from build123d import *

# Parameters (mm, degrees)
SKETCH_1_W          = 195
SKETCH_1_H          = 50
EXTRUDE_1_DEPTH     = 4
SKETCH_5_W          = 195
SKETCH_5_H          = 50
EXTRUDE_2_DEPTH     = 4
SKETCH_2_R          = 1.5
CUT_EXTRUDE_1_DEPTH = 124.074164633
SKETCH_4_W          = 20
SKETCH_4_H          = 14
CUT_EXTRUDE_3_DEPTH = 124.074164633
FILLET_1_R          = 1.5
SKETCH_6_W          = 23
SKETCH_6_H          = 23
CUT_EXTRUDE_4_DEPTH = 124.074164633
FILLET_2_R          = 5
SKETCH_7_W          = 15
SKETCH_7_H          = 15
EXTRUDE_3_DEPTH     = 4
SKETCH_3_R          = 1.5
CUT_EXTRUDE_2_DEPTH = 124.074164633
SKETCH_8_R          = 1.5
CUT_EXTRUDE_5_DEPTH = 124.074164633
SKETCH_9_W          = 165
SKETCH_9_H          = 13
CUT_EXTRUDE_6_DEPTH = 124.074164633
FILLET_3_R          = 20


with BuildPart() as part:
    # 草图1 → 凸台-拉伸1 (new body)
    with BuildSketch(Plane.XY):
        Rectangle(SKETCH_1_W, SKETCH_1_H)
    extrude(amount=EXTRUDE_1_DEPTH)

    # 草图5 → 凸台-拉伸2 (add)
    with BuildSketch(Plane.XY.offset(4)):
        with Locations((0, 50)):
            Rectangle(SKETCH_5_W, SKETCH_5_H)
    extrude(amount=-EXTRUDE_2_DEPTH)

    # 草图2 → 切除-拉伸1 (cut, through all)
    with BuildSketch(Plane.XY.offset(4)):
        with Locations((-47.5, -3)):
            Circle(SKETCH_2_R)
        with Locations((-47.5, 9)):
            Circle(SKETCH_2_R)
        with Locations((47.5, 9)):
            Circle(SKETCH_2_R)
        with Locations((47.5, -3)):
            Circle(SKETCH_2_R)
    extrude(amount=-CUT_EXTRUDE_1_DEPTH, mode=Mode.SUBTRACT)

    # 草图4 → 切除-拉伸3 (cut, through all)
    with BuildSketch(Plane.XY.offset(4)):
        with Locations((47.5, 25)):
            Rectangle(SKETCH_4_W, SKETCH_4_H)
        with Locations((-47.5, 25)):
            Rectangle(SKETCH_4_W, SKETCH_4_H)
    extrude(amount=-CUT_EXTRUDE_3_DEPTH, mode=Mode.SUBTRACT)

    # 圆角1
    fillet_1_edges = [part.edges().sort_by_distance(p)[0] for p in [
        (37.5, 18, 2),
        (37.5, 32, 2),
        (57.5, 32, 2),
        (57.5, 18, 2),
        (-57.5, 32, 2),
        (-37.5, 32, 2),
        (-37.5, 18, 2),
        (-57.5, 18, 2),
    ]]
    fillet(fillet_1_edges, radius=FILLET_1_R)

    # 草图6 → 切除-拉伸4 (cut, through all)
    with BuildSketch(Plane.XY.offset(4)):
        with Locations((-86, 63.5)):
            Rectangle(SKETCH_6_W, SKETCH_6_H)
        with Locations((86, 63.5)):
            Rectangle(SKETCH_6_W, SKETCH_6_H)
    extrude(amount=-CUT_EXTRUDE_4_DEPTH, mode=Mode.SUBTRACT)

    # 圆角2
    fillet_2_edges = [part.edges().sort_by_distance(p)[0] for p in [
        (-74.5, 52, 2),
        (74.5, 52, 2),
    ]]
    fillet(fillet_2_edges, radius=FILLET_2_R)

    # 草图7 → 凸台-拉伸3 (add)
    with BuildSketch(Plane.XY.offset(4)):
        with Locations((90, -32.5)):
            Rectangle(SKETCH_7_W, SKETCH_7_H)
        with Locations((-90, -32.5)):
            Rectangle(SKETCH_7_W, SKETCH_7_H)
    extrude(amount=-EXTRUDE_3_DEPTH)

    # 草图3 → 切除-拉伸2 (cut, through all)
    with BuildSketch(Plane.XY.offset(4)):
        with Locations((-90, 45)):
            Circle(SKETCH_3_R)
        with Locations((-90, -25)):
            Circle(SKETCH_3_R)
        with Locations((90, -25)):
            Circle(SKETCH_3_R)
        with Locations((90, 45)):
            Circle(SKETCH_3_R)
        with Locations((-90, 20)):
            Circle(SKETCH_3_R)
        with Locations((90, 20)):
            Circle(SKETCH_3_R)
    extrude(amount=-CUT_EXTRUDE_2_DEPTH, mode=Mode.SUBTRACT)

    # 草图8 → 切除-拉伸5 (cut, through all)
    with BuildSketch(Plane.XY.offset(4)):
        with Locations((0, 67.5)):
            Circle(SKETCH_8_R)
        with Locations((-60, 67.5)):
            Circle(SKETCH_8_R)
        with Locations(Location((60, 67.5, 0), (0, 0, 180))):
            Circle(SKETCH_8_R)
    extrude(amount=-CUT_EXTRUDE_5_DEPTH, mode=Mode.SUBTRACT)

    # 草图9 → 切除-拉伸6 (cut, through all)
    with BuildSketch(Plane.XY.offset(4)):
        with Locations((0, -18.5)):
            Rectangle(SKETCH_9_W, SKETCH_9_H)
    extrude(amount=-CUT_EXTRUDE_6_DEPTH, mode=Mode.SUBTRACT)

    # 圆角3
    fillet_3_edges = [part.edges().sort_by_distance(p)[0] for p in [
        (-82.5, -12, 2),
        (82.5, -12, 2),
    ]]
    fillet(fillet_3_edges, radius=FILLET_3_R)


solid = part.part
The model under review builds one solid part; all positions refer to its coordinate system, in mm. A direction names the side the tool comes from. Coordinates: 2 decimals unless noted, no trailing zeros. Loops run counter-clockwise (first coordinate to the right, second up) from the corner with the lowest first, then second, coordinate; pieces in that order, holes last. Notation, with made-up numbers: (27.5, 62.25) -> (46.5, 62.25) arc R11 ccw to (46.5, 75.25) -> close; hole circle Ø3 at (23, 14.5). An arc over 180 degrees is marked (long way). Use a Markdown table: item, result. Add a question column.
1. Add section A-A on y = -14. Write out the cut boundary in (x, z), plus the area to 3 significant figures.
2. Add section B-B on z = 2.3. Give the number of separate pieces and of enclosed holes in the cut face, plus the area to 3 significant figures.
3. To check wall thickness, follow line 1 (Y direction, x = 47.5, z = 2.6); line 2 (Y direction, x = -60, z = 2.7); line 3 (X direction, y = 8, z = 3.45). State the ranges of each line that lie inside material, in increasing order.
4. Add section C-C on x = 14.5. Write out the cut boundary in (y, z), plus the area to 3 significant figures.
5. Clearance check with flat-ended pins moving along their axes: pin 1 Ø1.2 at (y, z) = (68, 2) entering from +X; pin 2 Ø2 at (x, z) = (23.5, 1.5) entering from -Y. State where each tip first meets the part, or that it passes through.
6. Machinability: for faces 4 (the face through (88, 52, 2)), 5 (the face through (-37.5, 25, 2)), 6 (the face through (-1, -12, 2)), which of the approach directions +Z, -Z, +X, -X, +Y, -Y give a long, thin tool a straight path to every point of the face, cutting with its end or side? Answer none if there is none.
7. Draft analysis for pull direction Y (two halves, no side actions). For faces 1 (the face through (-1, 31, 4)), 2 (the face through (76.797, -18.014, 1.972)), 3 (the face through (-57.5, 25, 2)), state which applies: pulls with the +Y half, pulls with the -Y half, needs draft (parallel to the pull), parting line crosses it, or undercut.
Returned:
| question | item | result |
|---|---|---|
| 1 | outline | (-97.5, 0) -> (-71.22, 0) -> (-71.22, 4) -> (-97.5, 4) -> close; (71.22, 0) -> (97.5, 0) -> (97.5, 4) -> (71.22, 4) -> close |
| 1 | area | 210 mm² |
| 2 | separate pieces | 1 |
| 2 | enclosed holes | 15 |
| 2 | area | 16,300 mm² |
| 3 | line 1 | y = -12 to -4.5, -1.5 to 7.5, 10.5 to 18, 32 to 75 |
| 3 | line 2 | y = -12 to 66, 69 to 75 |
| 3 | line 3 | x = -97.5 to -48.62, -46.38 to 46.38, 48.62 to 97.5 |
| 4 | outline | (-12, 0) -> (75, 0) -> (75, 4) -> (-12, 4) -> close |
| 4 | area | 348 mm² |
| 5 | pin 1 | stops at x = 74.5 |
| 5 | pin 2 | stops at y = -12 |
| 6 | face 4 | +Z, -Z, +X, +Y |
| 6 | face 5 | +Z, -Z |
| 6 | face 6 | +Z, -Z, -Y |
| 7 | face 1 | needs draft |
| 7 | face 2 | pulls with the -Y half |
| 7 | face 3 | undercut |
